Verification items for the finished model (mm, model axes). A direction names the side the tool comes from. Coordinates: 2 decimals unless noted, no trailing zeros. Write each loop counter-clockwise with the first axis right and the second up, starting at its lowest first coordinate (ties: lowest second). Pieces come first, ordered by that corner, then holes. Notation, with made-up numbers: (70.5, -38.75) -> (76.5, -38.75) arc R19 ccw to (76.5, -26.75) -> close; hole circle Ø9 at (17, 70). An arc over 180 degrees is marked (long way). Write item = value, one per line. Start each with the question number.
(1) Section check B-B (y = 13.5). Record the cut outline in (x, z), plus the area to 3 significant figures.
(2) Set-up check for faces 1 (the face through (-4, 30, 4)), 2 (the face through (6, 2, -10)): record each of +Z, -Z, +X, -X, +Y, -Y from which the full face is reachable in a straight line by a thin tool's end or side.
(3) Section check D-D (z = 12.75). Record the cut outline in (x, y), plus the area to 3 significant figures.
(4) Material ranges on probe 1 along Y at (x, z) = (-2.75, 12); probe 2 along Z at (x, y) = (4, 20); probe 3 along X at (y, z) = (11.5, 6.25), recorded low to high. Write a range as [from, to].
(5) Section check A-A (x = 0). Record the cut outline in (y, z).
(6) Gauge pin test, flat ends, axial feed: pin 1 Ø10 at (x, z) = (-7.5, -1) entering from +Y; pin 2 Ø3 at (x, y) = (-1.5, 26) entering from -Z; pin 3 Ø1.5 at (x, y) = (-11.5, 10) entering from -Z; pin 4 Ø5 at (x, y) = (9, 21) entering from +Z. Record the tip position at first contact, or that the pin passes through.
(7) Section check C-C (x = -12). Record the cut outline in (y, z).
(8) Mould release check, pull along Z, two halves, no side actions. Record for faces 3 (the face through (3, 0, -10)), 4 (the face through (7.19, 14.79, 2.26)), 5 (the face through (7.98, 15.8, 2.51)): released by +Z, released by -Z, zero draft, split by the parting line, or undercut.
```python
from build123d import *

# Parameters (mm, degrees)
F2_R     = 6
F0_R     = 11
F6_R     = 15
F7_DEPTH = 2
F5_R     = 5
F4_R     = 10


with BuildPart() as f3:
    # F2 (on offset) → F3 section 0
    with BuildSketch(Plane.XZ.offset(-30)):
        Circle(F2_R)
    # F0 (on Front) → F3 section 1
    with BuildSketch(Plane.XZ):
        Circle(F0_R)
    loft()

    # F6 (on Front) → F7 (join)
    with BuildSketch(Plane.XZ):
        Circle(F6_R)
    extrude(amount=-F7_DEPTH)

    # F5 (on offset) → F8 section 0
    with BuildSketch(Plane.XZ.offset(-30)):
        Circle(F5_R)
    # F4 (on Front) → F8 section 1
    with BuildSketch(Plane.XZ):
        Circle(F4_R)
    loft(mode=Mode.SUBTRACT)


solid = f3.part
```
Response:
q1.outline = circle Ø17.5 at (0, 0); hole circle Ø15.5 at (0, 0)
q1.area = 51.8 mm2
q2.face_1 = +Z, -Z, +X, -X, +Y
q2.face_2 = +Y
q3.outline = (-7.9, 0) -> (7.9, 0) -> (7.9, 2) -> (-7.9, 2) -> close
q3.area = 31.6 mm2
q4.probe_1 = [0, 2]
q4.probe_2 = [-6.54, -5.33], [5.33, 6.54]
q4.probe_3 = [-6.59, -5.13], [5.13, 6.59]
q5.outline = (0, -15) -> (2, -15) -> (2, -10.67) -> (30, -6) -> (30, -5) -> (0, -10) -> close; (0, 10) -> (30, 5) -> (30, 6) -> (2, 10.67) -> (2, 15) -> (0, 15) -> close
q6.pin_1 = 30
q6.pin_2 = -6.84
q6.pin_3 = through
q6.pin_4 = 3.82
q7.outline = (0, -9) -> (2, -9) -> (2, 9) -> (0, 9) -> close
q8.face_3 = zero draft
q8.face_4 = undercut
q8.face_5 = split by the parting line
